Here's how the part is built. I have some questions about the finished solid (model axes, mm). A direction names the side the tool comes from. Coordinates: 2 decimals unless noted, no trailing zeros. Loops run counter-clockwise (first coordinate to the right, second up) from the corner with the lowest first, then second, coordinate; pieces in that order, holes last. Notation, with made-up numbers: (35, -8) -> (57, -8) arc R15 cw to (57, -4) -> close; hole circle Ø3 at (82, 25). An arc over 180 degrees is marked (long way). Answer as a JSON object with one key per item and string values. Group by question number.
1) I need wall thicknesses on probe 1 along Z at (x, y) = (145, -13); probe 2 along X at (y, z) = (-84, 20); probe 3 along Y at (x, z) = (141.5, 47). Which ranges of each line are inside material? Lowest first, please. Write a range as [from, to].
2) If we mould it in two halves opening along X, with no side actions, what happens to faces 1 (the flat face through (0, -77, 23)), 2 (the flat face through (51, -22, 40)), 3 (the cylindrical face through (130.015, -77.185, 20.66))? For each: +X half, -X half, draft (parallel to the pull), parting line (faces both ways), or undercut.
3) I want a section at B-B (z = 20). Write out the boundary of the cut face in (x, y), then the cut area to 3 significant figures.
4) I want a section at A-A (y = -74.5). Write out the boundary of the cut face in (x, z).
5) Which directions (+Z, -Z, +X, -X, +Y, -Y) give clear straight access to the entire face, cutting with the end or side of a thin tool? Please do faces 4 (the cylindrical face through (1, -43, 20)), 5 (the flat face through (126, -45, 57)), 6 (the cylindrical face through (52, -99, 38)), 7 (the cylindrical face through (102, -56, 93)).
6) I'm going to push a flat-ended pin straight in: pin 1 (12 mm diameter, centred on y = -82.5, z = 74, fed in from -X). Where does the tip first touch, or does it pass through?
7) I want a section at D-D (x = 141.5). Write out the boundary of the cut face in (y, z).
8) I want a section at C-C (x = 88). Write out the boundary of the cut face in (y, z).
```python
from build123d import *

# Parameters (mm, degrees)
F0_R     = 15
F1_DEPTH = 100
F3_DEPTH = 150
F5_R     = 5
F7_DEPTH = 300


# Not quite as in the source:
# - the program builds the solid bodies; features that only make, move or delete a surface that nothing else refers to are left out


with BuildPart() as f1:
    # F0 (on Front) → F1 (new body)
    with BuildSketch(Plane.XZ):
        Polygon((0, 40), (0, 0), (200, 0), (200, 150), (100, 150), (100, 40), align=None)
        with Locations((145, 20)):
            Circle(F0_R, mode=Mode.SUBTRACT)
    extrude(amount=F1_DEPTH)

    # F2 (on Top) → F3 (cut, through all)
    with BuildSketch(Plane.XY):
        with BuildLine():
            Line((-30, -55), (170, -55))
            ThreePointArc((170, -55), (175, -50), (170, -45))
            Line((170, -45), (-30, -45))
            Line((-30, -45), (-30, -55))
        make_face()
    extrude(amount=F3_DEPTH, mode=Mode.SUBTRACT)

    # F5
    f5_edges = [f1.edges().sort_by_distance(p)[0] for p in [
        (100, -45, 95),
        (100, -55, 95),
        (100, -100, 95),
        (50, -100, 40),
        (50, -55, 40),
        (50, -45, 40),
        (100, 0, 95),
        (50, 0, 40),
        (0, 0, 20),
        (0, -45, 20),
        (0, -22.5, 0),
        (0, -55, 20),
        (0, -100, 20),
        (0, -77.5, 0),
        (100, -22.5, 150),
        (100, -77.5, 150),
    ]]
    fillet(f5_edges, radius=F5_R)

    # F6 (on face) → F7 (cut)
    with BuildSketch(Plane.YZ.offset(200)):
        with BuildLine():
            Line((-45, -10), (-45, 120))
            ThreePointArc((-45, 120), (-50, 125), (-55, 120))
            Line((-55, 120), (-55, -10))
            Line((-55, -10), (-45, -10))
        make_face()
    extrude(amount=-F7_DEPTH, mode=Mode.SUBTRACT)


solid = f1.part
```
Determined:
{
 "1": {"probe 1": "[0, 5], [35, 150]", "probe 2": "[0, 130], [160, 200]", "probe 3": "[-100, -55], [-45, 0]"},
 "2": {"face 1": "-X half", "face 2": "draft", "face 3": "undercut"},
 "3": {"outline": "(0, -95) arc R5 ccw to (5, -100) -> (130, -100) -> (130, -55) -> (5, -55) arc R5 ccw to (0, -60) -> close; (0, -40) arc R5 ccw to (5, -45) -> (130, -45) -> (130, 0) -> (5, 0) arc R5 ccw to (0, -5) -> close; (160, -100) -> (200, -100) -> (200, -55) -> (160, -55) -> close; (160, -45) -> (200, -45) -> (200, 0) -> (160, 0) -> close", "area": "15,300 mm^2"},
 "4": {"outline": "(0, 5) arc R5 ccw to (5, 0) -> (200, 0) -> (200, 150) -> (105, 150) arc R5 ccw to (100, 145) -> (100, 40) -> (0, 40) -> close; hole circle Ø30 at (145, 20)"},
 "5": {"face 4": "+Z, -Z, -X", "face 5": "-Z, -X", "face 6": "+Z, -X, -Y", "face 7": "+Z, -X"},
 "6": {"pin 1": "x = 100"},
 "7": {"outline": "(-100, 0) -> (-55, 0) -> (-55, 5.41) -> (-100, 5.41) -> close; (-100, 34.59) -> (-55, 34.59) -> (-55, 150) -> (-100, 150) -> close; (-45, 0) -> (0, 0) -> (0, 5.41) -> (-45, 5.41) -> close; (-45, 34.59) -> (0, 34.59) -> (0, 150) -> (-45, 150) -> close"},
 "8": {"outline": "(-100, 0) -> (-55, 0) -> (-55, 35) arc R5 ccw to (-60, 40) -> (-95, 40) arc R5 ccw to (-100, 35) -> close; (-45, 0) -> (0, 0) -> (0, 35) arc R5 ccw to (-5, 40) -> (-40, 40) arc R5 ccw to (-45, 35) -> close"}
}
